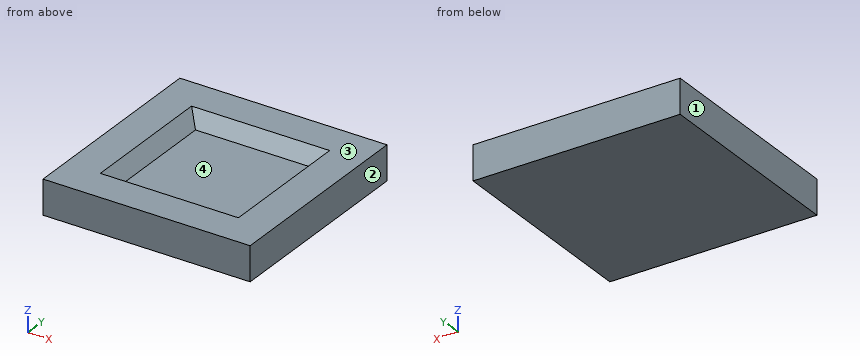
Autodesk Inventor part; units mm, degrees
sketch "Boceto1" plane through (0, 0, 0) normal (0, 0, 1) x (1, 0, 0)
  line L0 (-75, 75) -> (75, 75)
  line L1 (75, 75) -> (75, -75)
  line L2 (75, -75) -> (-75, -75)
  line L3 (-75, -75) -> (-75, 75)
  line L4 (-75, 75) -> (75, -75) construction
  line L5 (75, 75) -> (-75, -75) construction
  point P0 (0, 0)
  dimension "d0" = 150
  dimension "d1" = 150
extrude "Extrusión1" add sketch "Boceto1" along normal blind 25
sketch "Boceto2" plane through (0, 0, 25) normal (0, 0, 1) x (1, 0, 0)
  line L0 (-50, 50) -> (50, 50)
  line L1 (50, 50) -> (50, -50)
  line L2 (50, -50) -> (-50, -50)
  line L3 (-50, -50) -> (-50, 50)
  line L4 (-50, 50) -> (50, -50) construction
  line L5 (50, 50) -> (-50, -50) construction
  point P0 (0, 0)
  dimension "d4" = 100
  dimension "d5" = 100
ref_plane "Plano de trabajo1" through (0, 0, 15) normal (0, 0, 1) x (1, 0, 0)
sketch "Boceto4" plane through (0, 0, 15) normal (0, 0, 1) x (1, 0, 0)
  line L0 (-41.5714, 41.5714) -> (41.5714, 41.5714)
  line L1 (41.5714, 41.5714) -> (41.5714, -41.5714)
  line L2 (41.5714, -41.5714) -> (-41.5714, -41.5714)
  line L3 (-41.5714, -41.5714) -> (-41.5714, 41.5714)
  line L4 (-41.5714, 41.5714) -> (41.5714, -41.5714) construction
  line L5 (41.5714, 41.5714) -> (-41.5714, -41.5714) construction
  point P0 (0, 0)
  dimension "d9" = 83.1428
  dimension "d10" = 83.1428
loft "Solevación1" cut profiles "Boceto2", "Boceto4"
properties part number "Placa - Bolsillo 50°, Profundidad 10 mm"
Can you work these out from the model? Positions are in its coordinate system, mm. Face numbers are marked on the shaded views. Give positions to 0.01 mm unless a question says otherwise; leave off trailing zeros. Return JSON: item names as keys, results as strings.
Q1. I need wall thicknesses on probe 1 along Z at (x, y) = (36, 18); probe 2 along X at (y, z) = (20.5, 21); probe 3 along X at (y, z) = (-15, 20.5). Which ranges of each line are inside material? Lowest first, please.
Checks:
{"probe 1": "z = 0 to 15", "probe 2": "x = -75 to -46.63, 46.63 to 75", "probe 3": "x = -75 to -46.21, 46.21 to 75"}
Q2. We'd pull the mould along X, two halves only. Please class the marked faces 1, 2, 3 and 4: released by +X, released by -X, zero draft, split by the parting line, or undercut.
Checks:
{"face 1": "released by -X", "face 2": "released by +X", "face 3": "zero draft", "face 4": "undercut"}
Q3. For pin 1 Ø12 at (x, y) = (-5, 32) entering from +Z, with a flat end and sliding along its axis, tell me the tip position at first contact or that it passes through.
Checks:
{"pin 1": "stops at z = 15"}
